For this review, take the finished solid that the model builds, in its own axes (mm). Coordinates: 2 decimals unless noted, no trailing zeros. Loops run counter-clockwise (first coordinate to the right, second up) from the corner with the lowest first, then second, coordinate; pieces in that order, holes last. Notation, with made-up numbers: (42, -3) -> (99, -3) arc R13 cw to (99, 20) -> close; hole circle Ø10 at (9, 60.25). An arc over 180 degrees is marked (long way). Answer in a Markdown table with one row per item.
from build123d import *

# Parameters (mm, degrees)
SKETCH1_R                                      = 38.1
BOSS_EXTRUDE1_DEPTH                            = 6.35
CBORE_FOR_4_BUTTON_HEAD_CAP_SCREW1_D           = 2.8702
CBORE_FOR_4_BUTTON_HEAD_CAP_SCREW1_CBORE_D     = 4.826
CBORE_FOR_4_BUTTON_HEAD_CAP_SCREW1_CBORE_DEPTH = 1.905
CIRPATTERN1_COUNT                              = 8
SKETCH6_R                                      = 0.79375
CUT_EXTRUDE1_DEPTH                             = 55.254423783
CUT_EXTRUDE1_DEPTH_BACK                        = 55.254423783
SKETCH7_R                                      = 0.79375
CIRPATTERN2_COUNT                              = 12


with BuildPart() as part:
    # Sketch1 → Boss-Extrude1 (new body)
    with BuildSketch(Plane(origin=(0, 0, 0), x_dir=(1, 0, 0), z_dir=(0, 1, 0))):
        with Locations(Location((0, 0, 0), (0, 0, 270))):
            Circle(SKETCH1_R)
    extrude(amount=BOSS_EXTRUDE1_DEPTH)

    # CBORE for #4 Button Head Cap Screw1 (through all)
    with Locations(Plane(origin=(0, 0, 0), x_dir=(-1, 0, 0), z_dir=(0, -1, 0))):
        with Locations((0, -33.3375)):
            cbore_for_4_button_head_cap_screw1 = CounterBoreHole(CBORE_FOR_4_BUTTON_HEAD_CAP_SCREW1_D / 2, CBORE_FOR_4_BUTTON_HEAD_CAP_SCREW1_CBORE_D / 2, CBORE_FOR_4_BUTTON_HEAD_CAP_SCREW1_CBORE_DEPTH)

    # CirPattern1: CBORE for #4 Button Head Cap Screw1 ×8 about axis
    cirpattern1_axis = Axis((0, 0, 0), (0, 1, 0))
    for i in range(1, CIRPATTERN1_COUNT):
        add(cbore_for_4_button_head_cap_screw1.rotate(cirpattern1_axis, i * 360 / CIRPATTERN1_COUNT), mode=Mode.SUBTRACT)

    # Sketch6 → Cut-Extrude1 (cut, two sides)
    with BuildSketch(Plane(origin=(0, 6.35, 0), x_dir=(1, 0, 0), z_dir=(0, 1, 0))) as cut_extrude1_sk:
        with Locations(Location((0, 0, 0), (0, 0, 270))):
            Circle(SKETCH6_R)
    extrude(amount=CUT_EXTRUDE1_DEPTH, mode=Mode.SUBTRACT)
    extrude(cut_extrude1_sk.sketch, amount=-CUT_EXTRUDE1_DEPTH_BACK, mode=Mode.SUBTRACT)

    # Cut-Sweep1: sweep along a curve in space
    with BuildLine() as cut_sweep1_path:
        Line((0, 6.35, -15.875), (0, 0, -4.445))
    # Sketch7 → Cut-Sweep1 (sweep, cut)
    with BuildSketch(Plane(origin=(0, 6.35, 0), x_dir=(1, 0, 0), z_dir=(0, 1, 0))):
        with Locations((0, 15.875)):
            Circle(SKETCH7_R)
    cut_sweep1 = sweep(path=cut_sweep1_path.line, mode=Mode.SUBTRACT)

    # CirPattern2: Cut-Sweep1 ×12 about axis
    cirpattern2_axis = Axis((0, 6.35, 0), (0, 1, 0))
    for i in range(1, CIRPATTERN2_COUNT):
        add(cut_sweep1.rotate(cirpattern2_axis, i * 360 / CIRPATTERN2_COUNT), mode=Mode.SUBTRACT)


solid = part.part
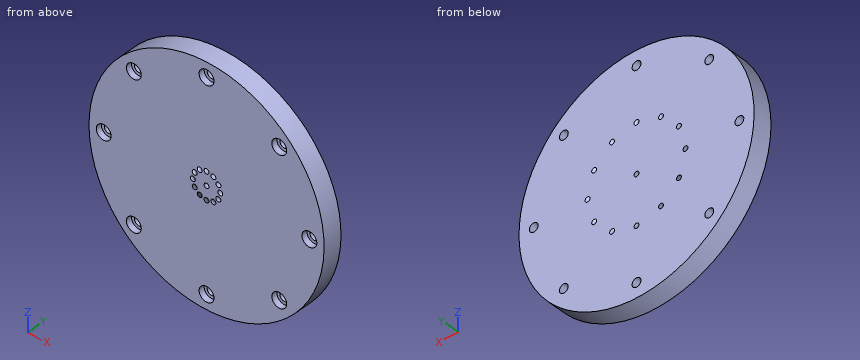
Item 1: Insertion check: pin 1 (2.5 mm diameter, centred on x = -1, z = 33.5, fed in from -Y) (3 decimals); pin 2 (2.5 mm diameter, centred on x = -23.57, z = 23.57, fed in from -Y); pin 3 (2 mm diameter, centred on y = 5.5, z = 17, fed in from -X); pin 4 (1.5 mm diameter, centred on y = 4.5, z = -1.5, fed in from -X). Each pin has a flat end and moves straight along its axis. Give the tip position at first contact, or say it passes through.
Worked answers:
| item | result |
|---|---|
| pin 1 | y = 1.905 |
| pin 2 | through |
| pin 3 | x = -34.58 |
| pin 4 | x = -38.09 |
Item 2: Take a section at B-B, the plane y = 5.25. Count the separate pieces of the cut face and the enclosed holes in it, and give its area (3 significant figures).
Worked answers:
| item | result |
|---|---|
| separate pieces | 1 |
| enclosed holes | 21 |
| area | 4,480 mm² |
Item 3: Take a section at A-A, the plane z = 19. State the section outline as (x, y) points, and give its area (3 significant figures).
Worked answers:
| item | result |
|---|---|
| outline | (-33.02, 0) -> (33.02, 0) -> (33.02, 6.35) -> (-33.02, 6.35) -> close |
| area | 419 mm² |
Item 4: For L1, parallel to Z at x = 1, y = 1.5; L2, parallel to Z at x = -22.5, y = 1.5; L3, parallel to X at y = 2.9, z = 0, list the stretches that pass through material, from the lowest coordinate up.
Worked answers:
| item | result |
|---|---|
| L1 | -38.09 to -35.53, -31.14 to 31.14, 35.53 to 38.09 |
| L2 | -30.75 to -25.73, -21.41 to 21.41, 25.73 to 30.75 |
| L3 | -38.1 to -34.77, -31.9 to -10.46, -8.87 to -0.79, 0.79 to 8.87, 10.46 to 31.9, 34.77 to 38.1 |
